Can you work these out from the model? Positions are in its coordinate system, mm. Give positions to 0.01 mm unless a question says otherwise; leave off trailing zeros. Order: outer loops, then holes, each group sorted by start corner. A loop starts at its lowest first (then second) coordinate and runs counter-clockwise, first axis right, second up. Notation, with made-up numbers: M 6.25,39 L 30.25,39 A19 ccw 30.25,58 Z; hole C -20.75,53 d9. An arc over 180 degrees is marked long. Answer as a JSON object with one key per item and string values.
```python
from build123d import *

# Parameters (mm, degrees)
CROQUIS1_R              = 7.5
SALIENTE_EXTRUIR1_DEPTH = 60
CHAFL_N2_SIZE           = 0.5
CHAFL_N2_SIZE_2         = 0.665279689


with BuildPart() as part:
    # Croquis1 → Saliente-Extruir1 (new body)
    with BuildSketch(Plane(origin=(0, 0, 0), x_dir=(1, 0, 0), z_dir=(0, 1, 0))):
        with Locations(Location((0, 0, 0), (0, 0, 270))):
            Circle(CROQUIS1_R)
    extrude(amount=SALIENTE_EXTRUIR1_DEPTH)

    # Cortar-Recubrir2: read off the stored shape, not the designer's step
    # Cortar-Recubrir2: loft between two sections, ruled curve by curve
    cortar_recubrir2_from = [
        Edge.make_bspline([(1.343543407, 40, -2.108291041), (-2.873038675, 40, -4.795377855), (-5.560125489, 40, -0.578795773), (-1.343543407, 40, 2.108291041), (2.873038675, 40, 4.795377855), (5.560125489, 40, 0.578795773), (1.343543407, 40, -2.108291041)], [0, 0, 0, 0, 0.5, 0.5, 0.5, 1, 1, 1, 1], 3, [1, 0.333333333, 0.333333333, 1, 0.333333333, 0.333333333, 1]),
    ]
    cortar_recubrir2_to = [
        Edge.make_bspline([(5.400627652, 60, 1.040779016), (7.482185685, 60, -9.760476288), (-3.319069619, 60, -11.842034321), (-5.400627652, 60, -1.040779016), (-7.482185685, 60, 9.760476288), (3.319069619, 60, 11.842034321), (5.400627652, 60, 1.040779016)], [0, 0, 0, 0, 0.5, 0.5, 0.5, 1, 1, 1, 1], 3, [1, 0.333333333, 0.333333333, 1, 0.333333333, 0.333333333, 1]),
    ]
    cortar_recubrir2 = Solid(Shell([*[Face.make_surface_from_curves(cortar_recubrir2_from[k], cortar_recubrir2_to[k]) for k in range(1)], Face(Wire(cortar_recubrir2_from)), Face(Wire(cortar_recubrir2_to))]))
    add(cortar_recubrir2, mode=Mode.SUBTRACT)

    # Chaflán1
    # the kernel refuses this chamfer: 0.665279689, 0.5 mm, written as the material it takes off along each edge
    with BuildSketch(Plane(origin=(0, 60, 0), x_dir=(0, 0, 1), z_dir=(-1, 0, 0))) as chafl_n1_piece_1:
        with BuildLine():
            Line((7.514142136, -0.514142136), (6.985857864, 0.014142136))
            Line((6.985857864, 0.014142136), (6.985857864, 0.024142136))
            ThreePointArc((6.985857864, 0.024142136), (7.242928932, 0.01), (7.5, 0.01))
            Line((7.5, 0.01), (7.51, 0))
            ThreePointArc((7.51, 0), (7.51, -0.257071068), (7.524142136, -0.514142136))
            Line((7.524142136, -0.514142136), (7.514142136, -0.514142136))
        make_face()
    revolve(axis=Axis((0, 60, 0), (0, 1, 0)), mode=Mode.SUBTRACT)
    with BuildSketch(Plane(origin=(0, 60, 0), x_dir=(0.9819323004404472, 1.2918958832590882e-15, 0.18923254834127032), z_dir=(-0.18923254834127032, 0, 0.9819323004404472))) as chafl_n1_piece_2:
        with BuildLine():
            Line((6.018807954, 0.018825944), (5.333201213, -0.667436596))
            Line((5.333201213, -0.667436596), (5.320226638, -0.664487154))
            ThreePointArc((5.320226638, -0.664487154), (5.410397761, -0.332303159), (5.487030093, 0.002969907))
            Line((5.487030093, 0.002969907), (5.5, 0.013305594))
            ThreePointArc((5.5, 0.013305594), (5.759403977, 0.013305594), (6.018807954, 0.032131538))
            Line((6.018807954, 0.032131538), (6.018807954, 0.018825944))
        make_face()
    revolve(axis=Axis((0, 60, 0), (0, 1, 0)), mode=Mode.SUBTRACT)

    # Simetría7: Cortar-Recubrir2 across plane
    add(cortar_recubrir2.mirror(Plane(origin=(0, 30, 0), x_dir=(0, 0, 1), z_dir=(0, -1, 0))), mode=Mode.SUBTRACT)

    # Chaflán2
    # the kernel refuses this chamfer: 0.665279689, 0.5 mm, written as the material it takes off along each edge
    with BuildSketch(Plane(origin=(0, 0, 0), x_dir=(0, 0, 1), z_dir=(-1, 0, 0))) as chafl_n2_piece_1:
        Polygon((7.5, CHAFL_N2_SIZE), (7.5 - CHAFL_N2_SIZE, 0), (7.5, 0), align=None)
    revolve(axis=Axis((0, 0, 0), (0, 1, 0)), mode=Mode.SUBTRACT)
    with BuildSketch(Plane(origin=(0, 0, 0), x_dir=(0.9819323004404472, 0, 0.18923254834127032), z_dir=(-0.18923254834127032, 0, 0.9819323004404472))) as chafl_n2_piece_2:
        with BuildLine():
            Line((5.5 + CHAFL_N2_SIZE_2, 0), (5.5 - CHAFL_N2_SIZE * 0.22264139859, CHAFL_N2_SIZE * 0.974900409085))
            ThreePointArc((5.5 - CHAFL_N2_SIZE * 0.22264139859, CHAFL_N2_SIZE * 0.974900409085), (5.442174309, 0.252877674), (5.5, 0))
            Line((5.5, 0), (5.5 + CHAFL_N2_SIZE_2, 0))
        make_face()
    revolve(axis=Axis((0, 0, 0), (0, 1, 0)), mode=Mode.SUBTRACT)


solid = part.part
```
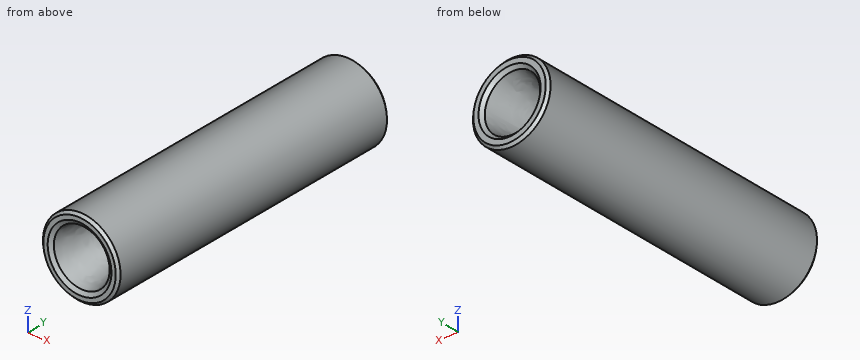
1) I'm going to push flat-ended pins straight in: pin 1 Ø2.5 at (x, z) = (1, 0.5) entering from +Y; pin 2 Ø1 at (x, y) = (5.5, 10.5) entering from +Z; pin 3 Ø6 at (y, z) = (22.5, 5) entering from +X. Where does each tip first touch, or does it pass through?
Results found:
{"pin 1": "stops at y = 40", "pin 2": "stops at z = 5.59", "pin 3": "stops at x = 7.23"}
2) I want a section at A-A on y = 37. Write out the boundary of the cut face in (x, z).
Results found:
{"outline": "C 0,0 d15"}
3) I need wall thicknesses on L1, parallel to X at y = 7, z = -3.25; L2, parallel to Z at x = 1, y = 11; L3, parallel to X at y = 43, z = -1.5. Which ranges of each line are inside material? Lowest first, please.
Results found:
{"L1": "x = -6.76 to -2.3, 2.3 to 6.76", "L2": "z = -7.43 to -3.09, 3.09 to 7.43", "L3": "x = -7.35 to -2.06, 2.06 to 7.35"}
